from build123d import *

# Parameters (mm, degrees)
F0_R     = 12.5
F1_DEPTH = 55
F2_SIZE  = 1
F4_D     = 14.75
F4_DEPTH = 27
F4_TIP   = 4.4313470653


with BuildPart() as f1:
    # F0 (on Top) → F1 (new body)
    with BuildSketch(Plane.XY):
        Circle(F0_R)
    extrude(amount=F1_DEPTH)

    # F2
    f2_edges = [f1.edges().sort_by_distance(p)[0] for p in [
        (-12.5, 0, 0),
        (-12.5, 0, 55),
    ]]
    chamfer(f2_edges, length=F2_SIZE)

    # F4
    with Locations(Plane.XY.offset(55)):
        with Locations((0, 0)):
            Hole(F4_D / 2, depth=F4_DEPTH)
            with Locations((0, 0, -(F4_DEPTH + F4_TIP / 2))):  # 118° drill point
                Cone(0, F4_D / 2, F4_TIP, mode=Mode.SUBTRACT)


solid = f1.part
Input: part model. Units: mm. Frame: model coordinates. A direction names the side the tool comes from. Round coordinates to 2 decimals unless told otherwise and drop trailing zeros. Order: outer loops, then holes, each group sorted by start corner. A loop starts at its lowest first (then second) coordinate and runs counter-clockwise, first axis right, second up.
1. Mould query, pull axis X, two halves, no side actions, for faces 1 (the face through (0, -8, 55)), 2 (the face through (1.183, -0.491, 24.338)), 3 (the face through (11.923, 3.755, 27.129)). Classes: released by +X, released by -X, zero draft, split by the parting line, or undercut.
The answers:
face 1: zero draft
face 2: undercut
face 3: split by the parting line
2. Cut plane B-B, the plane z = 10.5. Output: boundary loops of the cut face in (x, y), then the cut area to 3 significant figures.
The answers:
outline: circle Ø25 at (0, 0)
area: 491 mm2
3. Cut plane A-A, the plane z = 47.5. Output: boundary loops of the cut face in (x, y) (3 decimals).
The answers:
outline: circle Ø25 at (0, 0); hole circle Ø14.75 at (0, 0)
4. Set-up query: faces 4 (the face through (-7.034, 2.215, 41.311)), 5 (the face through (0, 0, 0)). Return all of +Z, -Z, +X, -X, +Y, -Y with unobstructed straight access to the full face (end or side cutting, diameter ignored); none if empty.
The answers:
face 4: +Z
face 5: -Z, +X, -X, +Y, -Y
5. Pin query (flat end, axial travel): P1, Ø3, axis at x = -2, z = 23.5, coming from the +Y side; P2, Ø10, axis at x = 7.5, z = 24, coming from the +Y side; P3, Ø10, axis at x = 7, z = 15.5, coming from the -Y side. Return the tip coordinate at first contact, or that it passes through.
The answers:
P1: stops at y = 12.49
P2: stops at y = 12.25
P3: stops at y = -12.34
6. Material intervals for line 1 (Y direction, x = 0, z = 43) (3 decimals); line 2 (Y direction, x = 2.5, z = 46.5); line 3 (X direction, y = -4.5, z = 31), sorted ascending.
The answers:
line 1: y = -12.5 to -7.375, 7.375 to 12.5
line 2: y = -12.25 to -6.94, 6.94 to 12.25
line 3: x = -11.66 to -5.84, 5.84 to 11.66
